```python
from build123d import *

# Parameters (mm, degrees)
F1_DEPTH = 17.5
F2_R     = 5
F3_W     = 40
F3_H     = 3
F4_DEPTH = 20


with BuildPart() as f1:
    # F0 (on Front) → F1 (new body, symmetric)
    with BuildSketch(Plane.XZ):
        Polygon((-25, 10), (0, 0), (0, 35), align=None)
    extrude(amount=F1_DEPTH, both=True)

    # F2
    f2_edges = [f1.edges().sort_by_distance(p)[0] for p in [
        (-12.5, -17.5, 22.5),
        (-12.5, -17.5, 5),
        (-12.5, 17.5, 22.5),
        (-12.5, 17.5, 5),
    ]]
    fillet(f2_edges, radius=F2_R)

    # F3 (on Front) → F4 (cut, symmetric)
    with BuildSketch(Plane.XZ):
        with Locations((-25, 10.642857)):
            Rectangle(F3_W, F3_H)
    extrude(amount=F4_DEPTH, both=True, mode=Mode.SUBTRACT)


solid = f1.part
```
Verification items for the finished model (mm, model axes). A direction names the side the tool comes from. Give positions to 0.01 mm unless a question says otherwise; leave off trailing zeros. Order: outer loops, then holes, each group sorted by start corner. A loop starts at its lowest first (then second) coordinate and runs counter-clockwise, first axis right, second up. Notation, with made-up numbers: M 25.25,41 L 58.25,41 A35 cw 58.25,73 Z; hole C 52.25,61 d2. An arc over 180 degrees is marked long. Answer in a Markdown table with one row per item. Add a question column.
Item 1: Tool access check on faces 1 (the flat face through (-5, 0, 11)), 2 (the flat face through (0, 0, 17)). Record the directions out of +Z, -Z, +X, -X, +Y, -Y that give a thin tool (end or side, any length) a straight path to the whole face; none if there is none.
Item 2: Gauge pin test, flat ends, axial feed: pin 1 (9 mm diameter, centred on x = -11, y = 7, fed in from -Z); pin 2 (3 mm diameter, centred on x = -20, z = 15, fed in from +Y); pin 3 (12 mm diameter, centred on y = 4, z = 30.5, fed in from -X). Record the tip position at first contact, or that the pin passes through.
Item 3: Section check B-B, the plane y = 13.5. Enter the section's corners in (x, z), and give its area (3 significant figures).
Item 4: Section check A-A, the plane y = -0.5. Enter the section's corners in (x, z).
Item 5: Scan lines: probe 1 along Z at (x, y) = (-19.5, 6); probe 2 along Z at (x, y) = (-13, 1); probe 3 along X at (y, z) = (5, 11.5). Record each from-to range of solid material in increasing order. Write a range as from..to.
Item 6: Mould release check, pull along Z, two halves, no side actions. Record for faces 3 (the flat face through (-14, 0, 12.143)), 4 (the cylindrical face through (-10.58, -16, 22.4)), 5 (the flat face through (-4, 17.5, 17)), 6 (the flat face through (-14, 0, 9.143)): released by +Z, released by -Z, zero draft, split by the parting line, or undercut.
Filled sheet:
| question | item | result |
|---|---|---|
| 1 | face 1 | -X, +Y, -Y |
| 1 | face 2 | +Z, -Z, +X, +Y, -Y |
| 2 | pin 1 | stops at z = 2.6 |
| 2 | pin 2 | stops at y = 16.07 |
| 2 | pin 3 | stops at x = -10.5 |
| 3 | outline | M -22.71,12.14 L -5,12.14 L -5,9.14 L -22.59,9.14 L 0,0.11 L 0,34.86 Z |
| 3 | area | 375 mm^2 |
| 4 | outline | M -22.86,9.14 L 0,0 L 0,35 L -22.86,12.14 L -5,12.14 L -5,9.14 Z |
| 5 | probe 1 | z = 7.8..9.14, 12.14..15.5 |
| 5 | probe 2 | z = 5.2..9.14, 12.14..22 |
| 5 | probe 3 | x = -5..0 |
| 6 | face 3 | undercut |
| 6 | face 4 | released by +Z |
| 6 | face 5 | zero draft |
| 6 | face 6 | undercut |
